Work out the finished part from the listing and answer in its coordinate system (mm). A direction names the side the tool comes from. Coordinates: 2 decimals unless noted, no trailing zeros. Order: outer loops, then holes, each group sorted by start corner. A loop starts at its lowest first (then second) coordinate and runs counter-clockwise, first axis right, second up. Notation, with made-up numbers: M 76.5,43 L 97.5,43 A24 cw 97.5,65 Z; hole C 27,-5 d2. An arc over 180 degrees is marked long. Use a Markdown table: item, result.
from build123d import *

# Parameters (mm, degrees)
F1_DEPTH = 15
F2_R     = 10
F4_D     = 8.1
F5_W     = 2
F5_H     = 7.5
F6_DEPTH = 15.001


with BuildPart() as f1:
    # F0 (on Top) → F1 (new body)
    with BuildSketch(Plane.XY):
        with BuildLine():
            Line((25.625, -30), (25.625, 30))
            Line((25.625, 30), (-11.742684, 30))
            ThreePointArc((-11.742684, 30), (-23.425524, 22.116407), (-30.625, 10))
            Line((-30.625, 10), (-58.590729, 10))
            ThreePointArc((-58.590729, 10), (-69.554492, 24.494897), (-86.875, 30))
            Line((-86.875, 30), (-108.125, 30))
            Line((-108.125, 30), (-108.125, -30))
            Line((-108.125, -30), (-86.875, -30))
            ThreePointArc((-86.875, -30), (-71.638705, -25.842897), (-60.625, -14.523688))
            Line((-60.625, -14.523688), (-60.625, -10))
            Line((-60.625, -10), (-58.590729, -10))
            Line((-58.590729, -10), (-30.625, -10))
            ThreePointArc((-30.625, -10), (-23.425524, -22.116407), (-11.742684, -30))
            Line((-11.742684, -30), (25.625, -30))
        make_face()
        with BuildLine():
            ThreePointArc((-20.472924, 2.5), (1.252311, 20.586946), (20.625, 0))
            ThreePointArc((20.625, 0), (1.252311, -20.586946), (-20.472924, -2.5))
            Line((-20.472924, -2.5), (-70.818459, -2.5))
            ThreePointArc((-70.818459, -2.5), (-103.125, 0), (-70.818459, 2.5))
            Line((-70.818459, 2.5), (-20.472924, 2.5))
        make_face(mode=Mode.SUBTRACT)
        with BuildLine():
            ThreePointArc((25.625, -30), (30.23108, 0), (25.625, 30))
            Line((25.625, 30), (25.625, -30))
        make_face()
        with BuildLine():
            ThreePointArc((-60.625, -14.523688), (-59.514214, -12.303958), (-58.590729, -10))
            Line((-58.590729, -10), (-60.625, -10))
            Line((-60.625, -10), (-60.625, -14.523688))
        make_face()
        with BuildLine():
            Line((-108.125, -30), (-108.125, 30))
            ThreePointArc((-108.125, 30), (-112.73108, 0), (-108.125, -30))
        make_face()
    extrude(amount=F1_DEPTH)

    # F2
    f2_edges = [f1.edges().sort_by_distance(p)[0] for p in [
        (-108.125, -30, 7.5),
        (-108.125, 30, 7.5),
        (25.625, 30, 7.5),
        (25.625, -30, 7.5),
        (-20.472924, -2.5, 7.5),
        (-20.472924, 2.5, 7.5),
        (-70.818459, 2.5, 7.5),
        (-70.818459, -2.5, 7.5),
        (-58.590729, -10, 7.5),
        (-30.625, -10, 7.5),
        (-30.625, 10, 7.5),
        (-58.590729, 10, 7.5),
    ]]
    fillet(f2_edges, radius=F2_R)

    # F4 (through all)
    with Locations(Plane.XZ.offset(10)):
        with Locations((-44.70608, 7.5)):
            Hole(F4_D / 2)

    # F5 (on face) → F6 (cut, through all)
    with BuildSketch(Plane.XY.offset(15)):
        with Locations((-44.70608, -6.25)):
            Rectangle(F5_W, F5_H)
    extrude(amount=-F6_DEPTH, mode=Mode.SUBTRACT)


solid = f1.part
(1) A cutting plane is placed at A-A (y = 5). Determine the outline of the cut face in (x, z), then the cut area to 3 significant figures.
Conclusion:
| item | result |
|---|---|
| outline | M -112.61,0 L -102.34,0 L -102.34,15 L -112.61,15 Z; M -70.41,0 L -21.34,0 L -21.34,15 L -70.41,15 Z; M 20.01,0 L 30.11,0 L 30.11,15 L 20.01,15 Z; hole C -44.71,7.5 d8.1 |
| area | 990 mm2 |
(2) A cutting plane is placed at B-B (x = 7.5). Determine the outline of the cut face in (y, z), then the cut area to 3 significant figures.
Conclusion:
| item | result |
|---|---|
| outline | M -30,0 L -19.21,0 L -19.21,15 L -30,15 Z; M 19.21,0 L 30,0 L 30,15 L 19.21,15 Z |
| area | 324 mm2 |
(3) Given P1, Ø1.1, axis at y = -6.5, z = 2, coming from the -X side; P2, Ø2, axis at x = -48.5, z = 7.5, coming from the -Y side; P3, Ø3, axis at y = -5, z = 1, coming from the +X side, each flat-ended and moving along its own axis, determine where each tip first touches the part or whether it passes through.
Conclusion:
| item | result |
|---|---|
| P1 | x = -112.55 |
| P2 | y = -10 |
| P3 | x = 30.17 |
(4) A cutting plane is placed at C-C (y = -24.5). Determine the outline of the cut face in (x, z), then the cut area to 3 significant figures.
Conclusion:
| item | result |
|---|---|
| outline | M -109.41,0 L -69.56,0 L -69.56,15 L -109.41,15 Z; M -20.92,0 L 26.91,0 L 26.91,15 L -20.92,15 Z |
| area | 1,320 mm2 |
(5) Which of the six approach directions +Z, -Z, +X, -X, +Y, -Y give full straight-line access (tool end or side, diameter ignored) to faces 1 (the flat face through (-50, 2.5, 7)), 2 (the cylindrical face through (-21.249, 24.215, 7.395)), 3 (the cylindrical face through (-40.657, -6.197, 7.575))?
Conclusion:
| item | result |
|---|---|
| face 1 | +Z, -Z |
| face 2 | +Z, -Z, +Y |
| face 3 | +Y, -Y |
(6) Straight lines are drawn through the part: L1, parallel to X at y = -7, z = 1.5; L2, parallel to Y at x = -50, z = 2.5; L3, parallel to X at y = 8.5, z = 12.5. For each, find the intervals that lie inside material, in ascending order.
Conclusion:
| item | result |
|---|---|
| L1 | -112.49 to -101.54, -72.14 to -45.71, -43.71 to -19.61, 19.4 to 29.99 |
| L2 | -10 to -2.5, 2.5 to 10 |
| L3 | -112.37 to -100.72, -73.03 to -18.79, 18.79 to 29.87 |
(7) Determine the mould class of faces 4 (the flat face through (-55, -2.5, 7)), 5 (the flat face through (3, 30, 7)), 6 (the cylindrical face through (24.14, -27.88, 7.6)), 7 (the flat face through (-43.706, -6, 13)) for opening direction X: pulls with the +X half, pulls with the -X half, needs draft (parallel to the pull), parting line crosses it, or undercut.
Conclusion:
| item | result |
|---|---|
| face 4 | undercut |
| face 5 | needs draft |
| face 6 | pulls with the +X half |
| face 7 | undercut |
